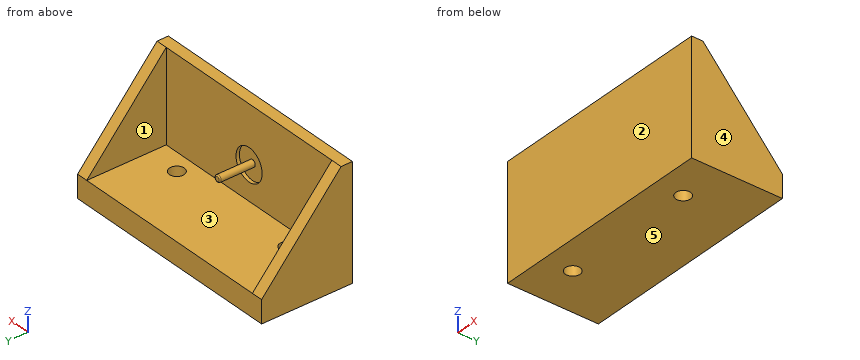
from build123d import *

# Parameters (mm, degrees)
SKETCH1_W               = 100
SKETCH1_H               = 50
BOSS_EXTRUDE1_DEPTH     = 5
SKETCH2_W               = 100
SKETCH2_H               = 10
BOSS_EXTRUDE2_DEPTH     = 40
CUT_EXTRUDE1_DEPTH      = 76.498344353
CUT_EXTRUDE1_DEPTH_BACK = 76.498344353
SKETCH4_3_R             = 3.25
CUT_EXTRUDE2_DEPTH      = 76.498344353
CUT_EXTRUDE2_DEPTH_BACK = 76.498344353
SKETCH4_R               = 3.25
BOSS_EXTRUDE5_DEPTH     = 5
SKETCH9_R               = 7.1
CUT_EXTRUDE3_DEPTH      = 1.5
SKETCH10_R              = 1.5
BOSS_EXTRUDE6_DEPTH     = 15.5
FILLET1_R               = 0.5


with BuildPart() as part:
    # Sketch1 → Boss-Extrude1 (new body)
    with BuildSketch(Plane(origin=(0, 0, 0), x_dir=(1, 0, 0), z_dir=(0, 1, 0))):
        Rectangle(SKETCH1_W, SKETCH1_H)
    extrude(amount=BOSS_EXTRUDE1_DEPTH)

    # Sketch2 → Boss-Extrude2 (add)
    with BuildSketch(Plane(origin=(0, 0, 0), x_dir=(1, 0, 0), z_dir=(0, 1, 0))):
        with Locations((0, 20)):
            Rectangle(SKETCH2_W, SKETCH2_H)
    extrude(amount=BOSS_EXTRUDE2_DEPTH)

    # Sketch4_3 → Cut-Extrude1 (cut, two sides: drawn at the far end of the back side and taken through both)
    with BuildSketch(Plane.XY.offset(-15).offset(-CUT_EXTRUDE1_DEPTH_BACK)):
        with Locations((-30, 12.5)):
            Circle(SKETCH4_3_R)
    extrude(amount=CUT_EXTRUDE1_DEPTH + CUT_EXTRUDE1_DEPTH_BACK, mode=Mode.SUBTRACT)

    # Sketch4 → Cut-Extrude2 (cut, two sides: drawn at the far end of the back side and taken through both)
    with BuildSketch(Plane.XY.offset(-15).offset(-CUT_EXTRUDE2_DEPTH_BACK)):
        with Locations(Location((30, 12.5, 0), (0, 0, 180))):
            Circle(SKETCH4_R)
    extrude(amount=CUT_EXTRUDE2_DEPTH + CUT_EXTRUDE2_DEPTH_BACK, mode=Mode.SUBTRACT)

    # Sketch8 → Boss-Extrude5 (add)
    with BuildSketch(Plane(origin=(50, 0, 0), x_dir=(0, 0, -1), z_dir=(1, 0, 0))):
        Polygon((15, 40), (15, 5), (-25, 5), align=None)
    boss_extrude5 = extrude(amount=-BOSS_EXTRUDE5_DEPTH)

    # Mirror1: Boss-Extrude5 across plane
    add(boss_extrude5.mirror(Plane(origin=(0, 0, 0), x_dir=(0, 0, 1), z_dir=(1, 0, 0))))

    # Sketch9 → Cut-Extrude3 (cut)
    with BuildSketch(Plane(origin=(0, 5, 0), x_dir=(1, 0, 0), z_dir=(0, 1, 0))):
        with Locations(Location((0, 0, 0), (0, 0, 270))):
            Circle(SKETCH9_R)
    extrude(amount=-CUT_EXTRUDE3_DEPTH, mode=Mode.SUBTRACT)

    # Sketch10 → Boss-Extrude6 (add)
    with BuildSketch(Plane(origin=(0, 3.5, 0), x_dir=(1, 0, 0), z_dir=(0, 1, 0))):
        with Locations(Location((0, 0, 0), (0, 0, 270))):
            Circle(SKETCH10_R)
    extrude(amount=BOSS_EXTRUDE6_DEPTH)

    # Fillet1
    fillet1_edges = [part.edges().sort_by_distance(p)[0] for p in [
        (0, 19, -1.5),
    ]]
    fillet(fillet1_edges, radius=FILLET1_R)


solid = part.part
Read the model definition and answer for the solid it produces. Units are mm, in the model's axes. Face numbers are marked on the shaded views. A direction names the side the tool comes from. Round coordinates to 2 decimals unless told otherwise and drop trailing zeros. Order: outer loops, then holes, each group sorted by start corner. A loop starts at its lowest first (then second) coordinate and runs counter-clockwise, first axis right, second up.
1) The part is cut by section B-B on z = -16.5. Write down the section's boundary in (x, y), plus the area to 3 significant figures.
2) Straight lines are drawn through the part: L1, parallel to X at y = 4.05, z = 0; L2, parallel to Y at x = -30, z = -20.25; L3, parallel to X at y = 7, z = -3. For each, find the intervals that lie inside material, in ascending order.
3) For the marked faces 1 and 2, determine the directions among +Z, -Z, +X, -X, +Y, -Y from which every point of the face is accessible in a straight line to the end or side of a thin tool.
4) Flat-ended cylindrical pins translate along their axes: pin 1 (6 mm diameter, centred on x = -39.5, z = 14.5, fed in from +Y); pin 2 (7 mm diameter, centred on x = -2, z = -3.5, fed in from +Y); pin 3 (7.5 mm diameter, centred on x = -30, y = 12.5, fed in from +Z). Find the tip coordinate at first contact, or state that the pin passes through.
5) The part is cut by section D-D on x = 0. Write down the section's boundary in (y, z), plus the area to 3 significant figures.
6) The mould has two halves that part along X. Classify the marked faces 3, 4 and 5: released by +X, released by -X, zero draft, split by the parting line, or undercut.
7) The part is cut by section C-C on y = 12.5. Write down the section's boundary in (x, z).
8) The part is cut by section A-A on x = 30. Write down the section's boundary in (y, z).
Resolved:
1. outline: (-50, 0) - (50, 0) - (50, 40) - (-50, 40) - close; hole circle Ø6.5 at (-30, 12.5); hole circle Ø6.5 at (30, 12.5)
1. area: 3,930 mm2
2. L1: x = -50 to -7.1, -1.5 to 1.5, 7.1 to 50
2. L2: y = 0 to 9.25, 15.75 to 40
2. L3: x = -50 to -45, 45 to 50
3. face 1: +Z, +Y
3. face 2: +Z, -Z, +X, -X, -Y
4. pin 1: stops at y = 5
4. pin 2: stops at y = 19
4. pin 3: stops at z = -15
5. outline: (0, -25) - (40, -25) - (40, -15) - (5, -15) - (5, -7.1) - (3.5, -7.1) - (3.5, -1.5) - (18.5, -1.5) arc R0.5 ccw to (19, -1) - (19, 1) arc R0.5 ccw to (18.5, 1.5) - (3.5, 1.5) - (3.5, 7.1) - (5, 7.1) - (5, 25) - (0, 25) - close
5. area: 625 mm2
6. face 3: undercut
6. face 4: released by +X
6. face 5: zero draft
7. outline: (-50, -25) - (-33.25, -25) - (-33.25, -15) - (-45, -15) - (-45, 16.43) - (-50, 16.43) - close; (-26.75, -25) - (26.75, -25) - (26.75, -15) - (-26.75, -15) - close; circle Ø3 at (0, 0); (33.25, -25) - (50, -25) - (50, 16.43) - (45, 16.43) - (45, -15) - (33.25, -15) - close
8. outline: (0, -25) - (9.25, -25) - (9.25, -15) - (5, -15) - (5, 25) - (0, 25) - close; (15.75, -25) - (40, -25) - (40, -15) - (15.75, -15) - close
